```python
from build123d import *

# Parameters (mm, degrees)
ESBO_O1_R                = 11
RESSALTO_EXTRUS_O1_DEPTH = 30
CASCA1_T                 = -2
FILETE1_R                = 1


with BuildPart() as part:
    # Esboço1 → Ressalto-extrusão1 (new body)
    with BuildSketch(Plane(origin=(0, 0, 0), x_dir=(1, 0, 0), z_dir=(0, 1, 0))):
        with Locations(Location((0, 0, 0), (0, 0, 270))):  # turned: the seam where the file's is
            Circle(ESBO_O1_R)
    extrude(amount=RESSALTO_EXTRUS_O1_DEPTH)

    # Casca1
    casca1_openings = [part.faces().sort_by_distance(p)[0] for p in [
        (0, 30, 0),
    ]]
    offset(amount=CASCA1_T, openings=casca1_openings, kind=Kind.INTERSECTION)

    # Filete1
    filete1_edges = [part.edges().sort_by_distance(p)[0] for p in [
        (0, 30, -11),
    ]]
    fillet(filete1_edges, radius=FILETE1_R)


solid = part.part
```
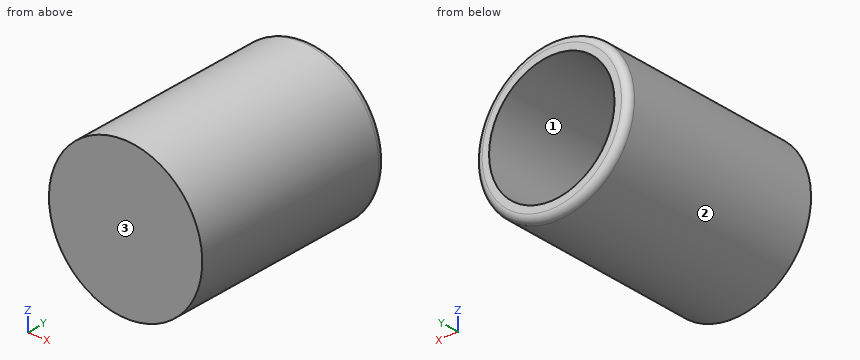
Geometry: final body of the model. Coordinates: model frame, mm. Face numbers are marked on the shaded views. Round coordinates to 2 decimals unless told otherwise and drop trailing zeros. Write each loop counter-clockwise with the first axis right and the second up, starting at its lowest first coordinate (ties: lowest second). Pieces come first, ordered by that corner, then holes. Notation, with made-up numbers: (-33.75, 81) -> (-4.75, 81) arc R10 ccw to (-4.75, 98) -> close; hole circle Ø9 at (-38, 8). An arc over 180 degrees is marked (long way). Return JSON: item names as keys, results as strings.
Q1. Ray query, line 1 (X direction, y = 24, z = 0); line 2 (Z direction, x = -0.75, y = 10.5); line 3 (Z direction, x = 7.75, y = 21.5). Return the intervals inside material, ascending.
From the geometry:
{"line 1": "-11 to -9, 9 to 11", "line 2": "-10.97 to -8.97, 8.97 to 10.97", "line 3": "-7.81 to -4.58, 4.58 to 7.81"}
Q2. Mould query, pull axis X, two halves, no side actions, for the marked faces 1, 2 and 3. Classes: +X half, -X half, draft (parallel to the pull), parting line (faces both ways), or undercut.
From the geometry:
{"face 1": "undercut", "face 2": "parting line", "face 3": "draft"}
Q3. Section B-B on y = 9.5. Return the cut outline in (x, z).
From the geometry:
{"outline": "circle Ø22 at (0, 0); hole circle Ø18 at (0, 0)"}
Q4. Section A-A on z = 0. Return the cut outline in (x, y), and give its area (3 significant figures).
From the geometry:
{"outline": "(-11, 0) -> (11, 0) -> (11, 29) arc R1 ccw to (10, 30) -> (9, 30) -> (9, 2) -> (-9, 2) -> (-9, 30) -> (-10, 30) arc R1 ccw to (-11, 29) -> close", "area": "156 mm2"}
Q5. First-contact query: pin 1 Ø5 at (y, z) = (10, -7.5) entering from +X; pin 2 Ø1.5 at (x, y) = (1, 9.5) entering from +Z; pin 3 Ø2 at (x, y) = (2.5, 24) entering from -Z. Flat tips, straight axial feed; report the tip coordinate or a pass-through.
From the geometry:
{"pin 1": "x = 9.8", "pin 2": "z = 11", "pin 3": "z = -10.9"}
Q6. Section C-C on x = 0. Return the cut outline in (y, z), and give its area (3 significant figures).
From the geometry:
{"outline": "(0, -11) -> (29, -11) arc R1 ccw to (30, -10) -> (30, -9) -> (2, -9) -> (2, 9) -> (30, 9) -> (30, 10) arc R1 ccw to (29, 11) -> (0, 11) -> close", "area": "156 mm2"}
